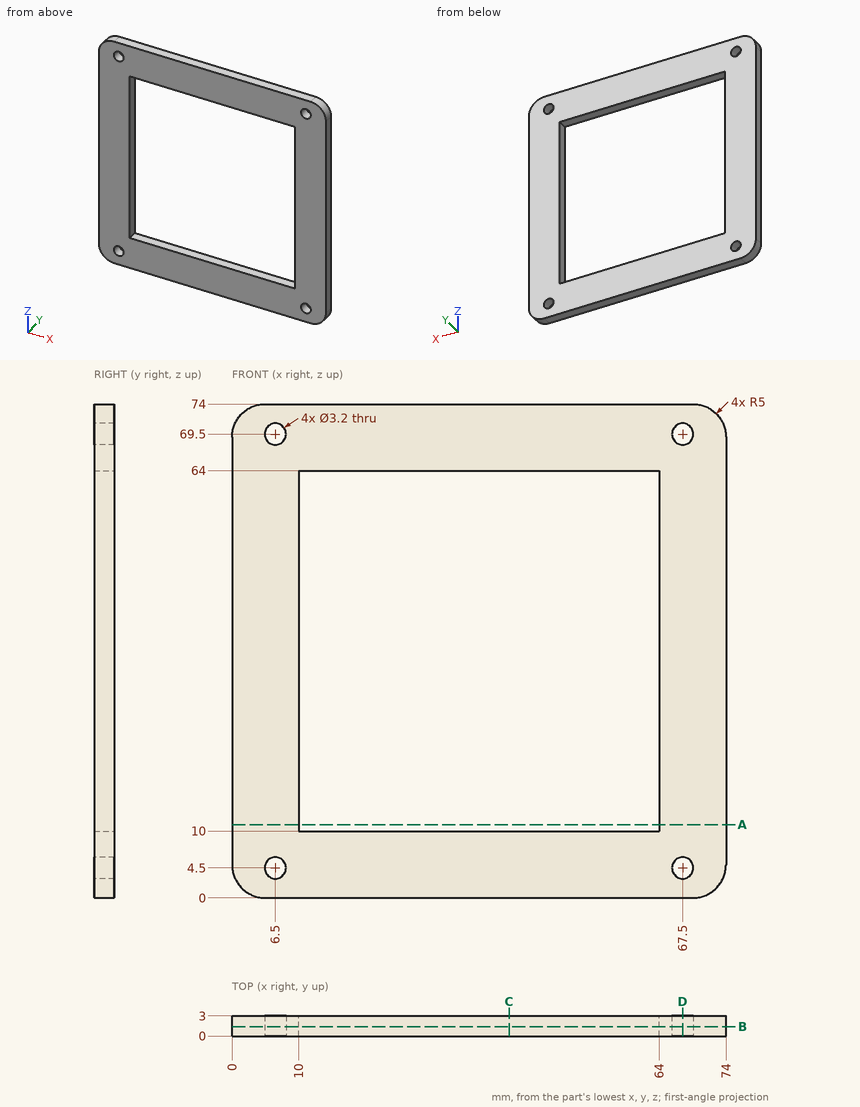
Design review of the part shown in the three views and the two pictorial views. Dimensions are in mm from the part's minimum x, y and z. Give positions to 0.01 mm unless a question says otherwise; leave off trailing zeros. Write each loop counter-clockwise with the first axis right and the second up, starting at its lowest first coordinate (ties: lowest second). Pieces come first, ordered by that corner, then holes.
(1) Wall thickness on line 1 along Z through (x, y) = (67.5, 1.9); line 2 along Z through (x, y) = (56, 2.3): over which ranges is each line inside the solid? List them lowest first.
Checked values:
line 1: z = 0 to 2.9, 6.1 to 67.9, 71.1 to 74
line 2: z = 0 to 10, 64 to 74
(2) Add section A-A (z = 11). Give the boundary of the cut face in (x, y), and give its area (3 significant figures).
Checked values:
outline: (0, 0) - (10, 0) - (10, 3) - (0, 3) - close; (64, 0) - (74, 0) - (74, 3) - (64, 3) - close
area: 60.0 mm2
(3) Clearance check with a flat-ended pin moving along its axis: pin 1 Ø3 at (x, z) = (67.5, 69.5) entering from -Y. State where the tip first meets the part, or that it passes through.
Checked values:
pin 1: passes through
(4) Add section C-C (x = 41.5). Give the boundary of the cut face in (y, z).
Checked values:
outline: (0, 0) - (3, 0) - (3, 10) - (0, 10) - close; (0, 64) - (3, 64) - (3, 74) - (0, 74) - close
(5) Add section D-D (x = 67.5). Give the boundary of the cut face in (y, z).
Checked values:
outline: (0, 0) - (3, 0) - (3, 2.9) - (0, 2.9) - close; (0, 6.1) - (3, 6.1) - (3, 67.9) - (0, 67.9) - close; (0, 71.1) - (3, 71.1) - (3, 74) - (0, 74) - close
(6) Add section B-B (y = 1.4). Give the boundary of the cut face in (x, z), and give its area (3 significant figures).
Checked values:
outline: (0, 5) arc R5 ccw to (5, 0) - (69, 0) arc R5 ccw to (74, 5) - (74, 69) arc R5 ccw to (69, 74) - (5, 74) arc R5 ccw to (0, 69) - close; hole circle Ø3.2 at (6.5, 4.5); hole circle Ø3.2 at (6.5, 69.5); hole (10, 10) - (64, 10) - (64, 64) - (10, 64) - close; hole circle Ø3.2 at (67.5, 4.5); hole circle Ø3.2 at (67.5, 69.5)
area: 2,510 mm2
